from build123d import *

# Parameters (mm, degrees)
F1_DEPTH = 450


with BuildPart() as f1:
    # F0 (on Front) → F1 (new body, symmetric)
    with BuildSketch(Plane.XZ):
        Polygon((-320, 0), (0, 0), (0, 230), (-320, 230), (-320, 460), (-640, 460), (-640, 690), (-960, 690), (-960, 920), (-1280, 920), (-1280, 1150), (-1600, 1150), (-1600, 920), align=None)
    extrude(amount=F1_DEPTH, both=True)


solid = f1.part
Here's how the part is built. I have some questions about the finished solid (model axes, mm). A direction names the side the tool comes from. Round coordinates to 2 decimals unless told otherwise and drop trailing zeros. Order: outer loops, then holes, each group sorted by start corner. A loop starts at its lowest first (then second) coordinate and runs counter-clockwise, first axis right, second up. Notation, with made-up numbers: (-7, -37.5) -> (0, -37.5) arc R20 ccw to (0, -18.5) -> close; hole circle Ø3 at (24.25, 66). An arc over 180 degrees is marked (long way). Return JSON: item names as keys, results as strings.
Q1. For pin 1 Ø1 at (y, z) = (178.5, 514) entering from +X; pin 2 Ø1.5 at (y, z) = (-263.5, 396) entering from +X; pin 3 Ø1.5 at (x, y) = (-624.5, -97.5) entering from -Z, each with a flat end and sliding along its axis, tell me the tip position at first contact or that it passes through.
Filled sheet:
{"pin 1": "stops at x = -640", "pin 2": "stops at x = -320", "pin 3": "stops at z = 218.32"}
Q2. I need wall thicknesses on line 1 along Z through (x, y) = (-223.5, -191.5); line 2 along X through (y, z) = (-78, 988.5); line 3 along X through (y, z) = (358, 818.5). Which ranges of each line are inside material? Lowest first, please. Write a range as from..to.
Filled sheet:
{"line 1": "z = 0..230", "line 2": "x = -1600..-1280", "line 3": "x = -1458.78..-960"}
Q3. If we section it at B-B on x = -278: List the corners of the cut face in (y, z) for me, plus the area to 3 significant figures.
Filled sheet:
{"outline": "(-450, 0) -> (450, 0) -> (450, 230) -> (-450, 230) -> close", "area": "207,000 mm^2"}
Q4. If we section it at A-A on y = -54: List the corners of the cut face in (x, z) for me.
Filled sheet:
{"outline": "(-1600, 920) -> (-320, 0) -> (0, 0) -> (0, 230) -> (-320, 230) -> (-320, 460) -> (-640, 460) -> (-640, 690) -> (-960, 690) -> (-960, 920) -> (-1280, 920) -> (-1280, 1150) -> (-1600, 1150) -> close"}
Q5. Which directions (+Z, -Z, +X, -X, +Y, -Y) give clear straight access to the entire face, cutting with the end or side of a thin tool? Please do faces 1 (the flat face through (-478, -6, 460)), 2 (the flat face through (-1600, -6, 1037)).
Filled sheet:
{"face 1": "+Z, +X, +Y, -Y", "face 2": "+Z, -Z, -X, +Y, -Y"}
Q6. If we section it at C-C on z = 1065: List the corners of the cut face in (x, y) for me, plus the area to 3 significant figures.
Filled sheet:
{"outline": "(-1600, -450) -> (-1280, -450) -> (-1280, 450) -> (-1600, 450) -> close", "area": "288,000 mm^2"}
